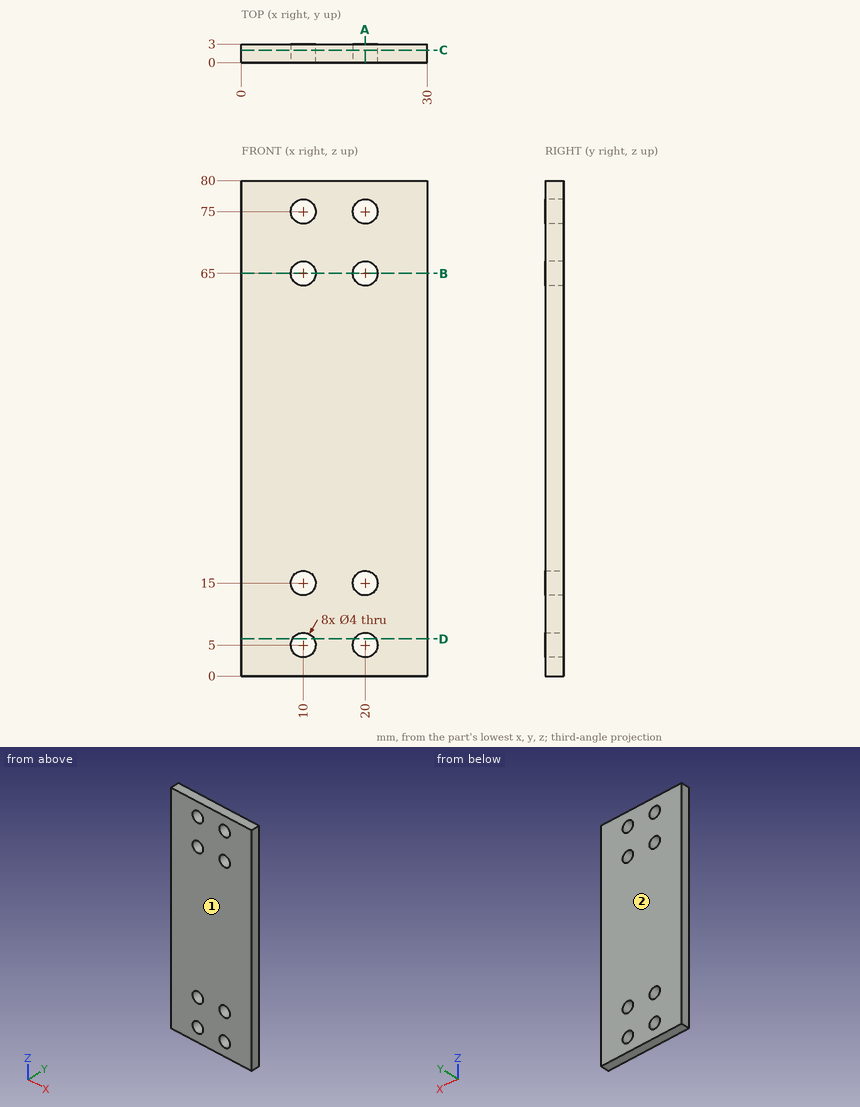
The drawing under review shows one solid part. Ordinate dimensions are in mm from its lowest x, y, z. Coordinates: 2 decimals unless noted, no trailing zeros. Loops run counter-clockwise (first coordinate to the right, second up) from the corner with the lowest first, then second, coordinate; pieces in that order, holes last.
Item 1: Draft analysis for pull direction Y (two halves, no side actions). For the marked faces 1 and 2, state which applies: pulls with the +Y half, pulls with the -Y half, needs draft (parallel to the pull), parting line crosses it, or undercut.
Completed:
face 1: pulls with the -Y half
face 2: pulls with the +Y half
Item 2: Add section D-D (z = 6). Write out the cut boundary in (x, y), and give its area (3 significant figures).
Completed:
outline: (0, 0) - (8.27, 0) - (8.27, 3) - (0, 3) - close; (11.73, 0) - (18.27, 0) - (18.27, 3) - (11.73, 3) - close; (21.73, 0) - (30, 0) - (30, 3) - (21.73, 3) - close
area: 69.2 mm2
Item 3: Clearance check with a flat-ended pin moving along its axis: pin 1 (3.5 mm diameter, centred on x = 20, z = 15, fed in from +Y). State where the tip first meets the part, or that it passes through.
Completed:
pin 1: passes through
Item 4: Wall thickness on L1, parallel to X at y = 2.15, z = 15; L2, parallel to Z at x = 20, y = 2.15; L3, parallel to Z at x = 8.25, y = 1.35: over which ranges is each line inside the solid? List them lowest first.
Completed:
L1: x = 0 to 8, 12 to 18, 22 to 30
L2: z = 0 to 3, 7 to 13, 17 to 63, 67 to 73, 77 to 80
L3: z = 0 to 4.03, 5.97 to 14.03, 15.97 to 64.03, 65.97 to 74.03, 75.97 to 80
Item 5: Add section C-C (y = 2). Give the number of separate pieces and of enclosed holes in the cut face, and give its area (3 significant figures).
Completed:
separate pieces: 1
enclosed holes: 8
area: 2,300 mm2
Item 6: Add section B-B (z = 65). Write out the cut boundary in (x, y), and give its area (3 significant figures).
Completed:
outline: (0, 0) - (8, 0) - (8, 3) - (0, 3) - close; (12, 0) - (18, 0) - (18, 3) - (12, 3) - close; (22, 0) - (30, 0) - (30, 3) - (22, 3) - close
area: 66.0 mm2
Item 7: Add section A-A (x = 20). Write out the cut boundary in (y, z), and give its area (3 significant figures).
Completed:
outline: (0, 0) - (3, 0) - (3, 3) - (0, 3) - close; (0, 7) - (3, 7) - (3, 13) - (0, 13) - close; (0, 17) - (3, 17) - (3, 63) - (0, 63) - close; (0, 67) - (3, 67) - (3, 73) - (0, 73) - close; (0, 77) - (3, 77) - (3, 80) - (0, 80) - close
area: 192 mm2
